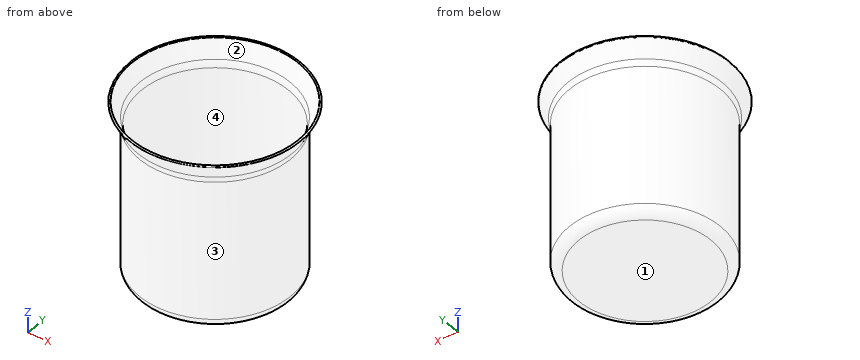
from build123d import *


with BuildPart() as f1:
    # F0 (on Right) → F1 (revolve)
    with BuildSketch(Plane.YZ):
        with BuildLine():
            Line((-70, 0), (0, 0))
            Line((0, 0), (0, 2))
            Line((0, 2), (-70, 2))
            ThreePointArc((-70, 2), (-75.656854, 4.343146), (-78, 10))
            Line((-78, 10), (-78, 156.45898))
            ThreePointArc((-78, 156.45898), (-78.454767, 160.36478), (-79.794738, 164.061611))
            Line((-79.794738, 164.061611), (-88.211146, 180.894427))
            ThreePointArc((-88.211146, 180.894427), (-89.552786, 181.341641), (-90, 180))
            Line((-90, 180), (-81.583592, 163.167184))
            ThreePointArc((-81.583592, 163.167184), (-80.401265, 159.905274), (-80, 156.45898))
            Line((-80, 156.45898), (-80, 10))
            ThreePointArc((-80, 10), (-77.071068, 2.928932), (-70, 0))
        make_face()
    revolve(axis=Axis((0, 0, 41.621631), (0, 0, 1)))


solid = f1.part
Source: CAD feature listing. Evaluate the final solid. Frame: model axes, mm. Face numbers are marked on the shaded views. Give positions to 0.01 mm unless a question says otherwise; leave off trailing zeros. Order: outer loops, then holes, each group sorted by start corner. A loop starts at its lowest first (then second) coordinate and runs counter-clockwise, first axis right, second up. Notation, with made-up numbers: (62, -18.5) -> (99, -18.5) arc R25 ccw to (99, 8.5) -> close; hole circle Ø3 at (79.25, 81). An arc over 180 degrees is marked (long way). Write item = value, one per line.
Q1. Material intervals for line 1 (X direction, y = 0, z = 119); line 2 (Z direction, x = 1.5, y = -3.5); line 3 (Y direction, x = -48, z = 142), sorted ascending. Write a range as from..to.
Data:
line_1 = -80..-78, 78..80
line_2 = 0..2
line_3 = -64..-61.48, 61.48..64
Q2. Pull-direction query (Y, two-part tool) for the marked faces 1, 2, 3 and 4; classes: released by +Y, released by -Y, zero draft, split by the parting line, or undercut.
Data:
face_1 = zero draft
face_2 = undercut
face_3 = split by the parting line
face_4 = undercut
Q3. Cut plane C-C, the plane z = 152. Output: boundary loops of the cut face in (x, y), and give its area (3 significant figures).
Data:
outline = circle Ø160 at (0, 0); hole circle Ø156 at (0, 0)
area = 993 mm^2
Q4. Cut plane A-A, the plane x = 0. Output: boundary loops of the cut face in (y, z).
Data:
outline = (-90, 180) -> (-81.58, 163.17) arc R15 cw to (-80, 156.46) -> (-80, 10) arc R10 ccw to (-70, 0) -> (70, 0) arc R10 ccw to (80, 10) -> (80, 156.46) arc R15 cw to (81.58, 163.17) -> (90, 180) arc R1 ccw to (88.21, 180.89) -> (79.79, 164.06) arc R17 ccw to (78, 156.46) -> (78, 10) arc R8 cw to (70, 2) -> (-70, 2) arc R8 cw to (-78, 10) -> (-78, 156.46) arc R17 ccw to (-79.79, 164.06) -> (-88.21, 180.89) arc R1 ccw to start
Q5. Pin query (flat end, axial travel): pin 1 (5 mm diameter, centred on x = -17.5, y = 29, fed in from +Z); pin 2 (3 mm diameter, centred on x = -51, y = 5, fed in from -Z); pin 3 (5 mm diameter, centred on y = 56.5, z = 137.5, fed in from +X); pin 4 (2 mm diameter, centred on x = 57.5, y = -49.5, fed in from +Z). Return the tip coordinate at first contact, or that it passes through.
Data:
pin_1 = 2
pin_2 = 0
pin_3 = 59.03
pin_4 = 5.9
